from build123d import *

# Parameters (mm, degrees)
SKETCH_1_W           = 100
SKETCH_1_H           = 50
EXTRUDE_1_DEPTH      = 25
SHELL_1_T            = -4
FILLET_1_R           = 4.5
SKETCH_2_R           = 0.75
CUT_EXTRUDE_1_DEPTH  = 5
CUT_EXTRUDE_3_DEPTH  = 2.5
SKETCH_8_W           = 36
SKETCH_8_H           = 12
CUT_EXTRUDE_4_DEPTH  = 3
SKETCH_9_W           = 42
SKETCH_9_H           = 21
CUT_EXTRUDE_7_DEPTH  = 2
SKETCH_7_W           = 1
SKETCH_7_H           = 42
CUT_EXTRUDE_8_DEPTH  = 1
SKETCH_11_W          = 1
SKETCH_11_H          = 21
CUT_EXTRUDE_10_DEPTH = 1
SKETCH_12_W          = 1
SKETCH_12_H          = 21
CUT_EXTRUDE_11_DEPTH = 1


with BuildPart() as part:
    # Sketch 1 → Extrude 1 (new body)
    with BuildSketch(Plane(origin=(0, 0, 0), x_dir=(1, 0, 0), z_dir=(0, 1, 0))):
        with Locations((50, -25)):
            Rectangle(SKETCH_1_W, SKETCH_1_H)
    extrude(amount=EXTRUDE_1_DEPTH)

    # Shell 1
    shell_1_openings = [part.faces().sort_by_distance(p)[0] for p in [
        (50, 25, 25),
    ]]
    offset(amount=SHELL_1_T, openings=shell_1_openings, kind=Kind.INTERSECTION)

    # Fillet 1
    fillet_1_edges = [part.edges().sort_by_distance(p)[0] for p in [
        (50, 0, 0),
        (100, 0, 25),
        (50, 0, 50),
        (0, 0, 25),
        (0, 12.5, 0),
        (100, 12.5, 0),
        (100, 12.5, 50),
        (0, 12.5, 50),
    ]]
    fillet(fillet_1_edges, radius=FILLET_1_R)

    # Sketch 2 → Cut-Extrude 1 (cut)
    with BuildSketch(Plane(origin=(0, 25, 0), x_dir=(1, 0, 0), z_dir=(0, 1, 0))):
        with Locations((6, -2)):
            Circle(SKETCH_2_R)
        with BuildLine():
            ThreePointArc((2, -5.25), (2.530330086, -5.469669914), (2.75, -6))
            Line((2.75, -6), (2.75, -2.75))
            Line((2.75, -2.75), (6, -2.75))
            ThreePointArc((6, -2.75), (5.469669914, -2.530330086), (5.25, -2))
            Line((5.25, -2), (2, -2))
            Line((2, -2), (2, -5.25))
        make_face()
        with Locations((2, -6)):
            Circle(SKETCH_2_R)
        with Locations(Location((94, -48, 0), (0, 0, 270))):
            Circle(SKETCH_2_R)
        with Locations(Location((94, -2, 0), (0, 0, 270))):
            Circle(SKETCH_2_R)
        with Locations((2, -44)):
            Circle(SKETCH_2_R)
        with BuildLine():
            Line((2.75, -47.25), (2.75, -44))
            ThreePointArc((2.75, -44), (2.530330086, -44.530330086), (2, -44.75))
            Line((2, -44.75), (2, -48))
            Line((2, -48), (5.25, -48))
            ThreePointArc((5.25, -48), (5.469669914, -47.469669914), (6, -47.25))
            Line((6, -47.25), (2.75, -47.25))
        make_face()
        with Locations((6, -48)):
            Circle(SKETCH_2_R)
    extrude(amount=-CUT_EXTRUDE_1_DEPTH, mode=Mode.SUBTRACT)

    # Sketch 2_6 → Cut-Extrude 3 (cut)
    with BuildSketch(Plane(origin=(0, 25, 0), x_dir=(1, 0, 0), z_dir=(0, 1, 0))):
        with BuildLine():
            Line((2.75, -44), (2.75, -6))
            ThreePointArc((2.75, -6), (2.530330086, -6.530330086), (2, -6.75))
            Line((2, -6.75), (2, -43.25))
            ThreePointArc((2, -43.25), (2.530330086, -43.469669914), (2.75, -44))
        make_face()
        with BuildLine():
            ThreePointArc((6.75, -2), (6.530330086, -2.530330086), (6, -2.75))
            Line((6, -2.75), (94, -2.75))
            ThreePointArc((94, -2.75), (93.469669914, -2.530330086), (93.25, -2))
            Line((93.25, -2), (6.75, -2))
        make_face()
        with BuildLine():
            Line((94, -47.25), (6, -47.25))
            ThreePointArc((6, -47.25), (6.530330086, -47.469669914), (6.75, -48))
            Line((6.75, -48), (93.25, -48))
            ThreePointArc((93.25, -48), (93.469669914, -47.469669914), (94, -47.25))
        make_face()
    extrude(amount=-CUT_EXTRUDE_3_DEPTH, mode=Mode.SUBTRACT)

    # Sketch 8 → Cut-Extrude 4 (cut)
    with BuildSketch(Plane.ZY.offset(-96)):
        with Locations((25, 14.5)):
            Rectangle(SKETCH_8_W, SKETCH_8_H)
    extrude(amount=-CUT_EXTRUDE_4_DEPTH, mode=Mode.SUBTRACT)

    # Sketch 9 → Cut-Extrude 7 (cut)
    with BuildSketch(Plane.ZY.offset(-96)):
        with Locations((25, 14.5)):
            Rectangle(SKETCH_9_W, SKETCH_9_H)
    extrude(amount=-CUT_EXTRUDE_7_DEPTH, mode=Mode.SUBTRACT)

    # Sketch 7 → Cut-Extrude 8 (cut)
    with BuildSketch(Plane(origin=(0, 4, 0), x_dir=(1, 0, 0), z_dir=(0, 1, 0))):
        with Locations((96, -25)):
            Rectangle(SKETCH_7_W, SKETCH_7_H)
    extrude(amount=-CUT_EXTRUDE_8_DEPTH, mode=Mode.SUBTRACT)

    # Sketch 11 → Cut-Extrude 10 (cut)
    with BuildSketch(Plane.XY.offset(4)):
        with Locations((96, 14.5)):
            Rectangle(SKETCH_11_W, SKETCH_11_H)
    extrude(amount=-CUT_EXTRUDE_10_DEPTH, mode=Mode.SUBTRACT)

    # Sketch 12 → Cut-Extrude 11 (cut)
    with BuildSketch(Plane(origin=(0, 0, 46), x_dir=(-1, 0, 0), z_dir=(0, 0, -1))):
        with Locations((-96, 14.5)):
            Rectangle(SKETCH_12_W, SKETCH_12_H)
    extrude(amount=-CUT_EXTRUDE_11_DEPTH, mode=Mode.SUBTRACT)


solid = part.part
Model file for the job. Use its own axes, mm. A direction names the side the tool comes from. Coordinates: 2 decimals unless noted, no trailing zeros. Order: outer loops, then holes, each group sorted by start corner. A loop starts at its lowest first (then second) coordinate and runs counter-clockwise, first axis right, second up. Notation, with made-up numbers: M 87,38 L 119,38 A14 ccw 119,51 Z; hole C -30,44 d9. An arc over 180 degrees is marked long. Return JSON: item names as keys, results as strings.
1. Saw through at C-C (x = 29). Give the cut face in (y, z).
Ans:
{"outline": "M 0,4.5 A4.5 ccw 4.5,0 L 25,0 L 25,2 L 22.5,2 L 22.5,2.75 L 25,2.75 L 25,4 L 4,4 L 4,46 L 25,46 L 25,47.25 L 22.5,47.25 L 22.5,48 L 25,48 L 25,50 L 4.5,50 A4.5 ccw 0,45.5 Z"}
2. Tool access for faces 1 (the face through (48, 24, 2.75)), 2 (the face through (99, 15, 25)), 3 (the face through (49, 15, 0)): list every direction of +Z, -Z, +X, -X, +Y, -Y with a clear straight run to the whole face (end or side of a thin tool).
Ans:
{"face 1": "+Y", "face 2": "none", "face 3": "-Z, +X, -X, +Y, -Y"}
3. Saw through at D-D (y = 6.25). Give the cut face in (x, z), and give its area (3 significant figures).
Ans:
{"outline": "M 0,4.5 A4.5 ccw 4.5,0 L 95.5,0 A4.5 ccw 100,4.5 L 100,45.5 A4.5 ccw 95.5,50 L 4.5,50 A4.5 ccw 0,45.5 Z; hole M 4,4 L 95.5,4 L 95.5,3 L 96.5,3 L 96.5,4 L 98,4 L 98,46 L 96.5,46 L 96.5,47 L 95.5,47 L 95.5,46 L 4,46 Z", "area": "1,030 mm^2"}
4. Saw through at A-A (y = 11.5). Give the cut face in (x, z).
Ans:
{"outline": "M 0,4.5 A4.5 ccw 4.5,0 L 95.5,0 A4.5 ccw 100,4.5 L 100,45.5 A4.5 ccw 95.5,50 L 4.5,50 A4.5 ccw 0,45.5 Z; hole M 4,4 L 95.5,4 L 95.5,3 L 96.5,3 L 96.5,4 L 98,4 L 98,7 L 99,7 L 99,43 L 98,43 L 98,46 L 96.5,46 L 96.5,47 L 95.5,47 L 95.5,46 L 4,46 Z"}
5. Flat gauge pins, fed straight in: pin 1 (2.5 mm diameter, centred on x = 6, z = 2, fed in from -Y); pin 2 (10 mm diameter, centred on x = 16, z = 36.5, fed in from +Y); pin 3 (1.1 mm diameter, centred on y = 3.5, z = 31, fed in from +X). Where does each tip first touch, or does it go through?
Ans:
{"pin 1": "y = 0.18", "pin 2": "y = 4", "pin 3": "x = 99.98"}
6. Pull direction X, two halves, no side cores. Call faces 4 (the face through (49, 0, 25)), 5 (the face through (98.647, 14.894, 48.717)), 6 (the face through (49, 24, 47.25)): +X half, -X half, draft (parallel to the pull), parting line (faces both ways), or undercut.
Ans:
{"face 4": "draft", "face 5": "+X half", "face 6": "undercut"}
7. Drill centre lines: probe 1 along Z at (x, y) = (6, 23.15); probe 2 along X at (y, z) = (5.5, 25). Where is each one in solid material? Low to high.
Ans:
{"probe 1": "0 to 1.25, 2.75 to 4, 46 to 47.25, 48.75 to 50", "probe 2": "0 to 4, 98 to 100"}
8. Saw through at B-B (z = 35). Give the cut face in (x, y).
Ans:
{"outline": "M 0,4.5 A4.5 ccw 4.5,0 L 95.5,0 A4.5 ccw 100,4.5 L 100,25 L 98,25 L 98,20.5 L 99,20.5 L 99,8.5 L 98,8.5 L 98,4 L 96.5,4 L 96.5,3 L 95.5,3 L 95.5,4 L 4,4 L 4,25 L 2.75,25 L 2.75,22.5 L 2,22.5 L 2,25 L 0,25 Z"}
